Build history of the part. All positions in model axes, mm. Face numbers are marked on the shaded views. A direction names the side the tool comes from. Coordinates: 2 decimals unless noted, no trailing zeros. Order: outer loops, then holes, each group sorted by start corner. A loop starts at its lowest first (then second) coordinate and runs counter-clockwise, first axis right, second up. Notation, with made-up numbers: (21, 57.25) - (27, 57.25) arc R31 ccw to (27, 95.25) - close; hole circle Ø2 at (26, 12). An arc over 180 degrees is marked (long way). Return JSON: item names as keys, results as strings.
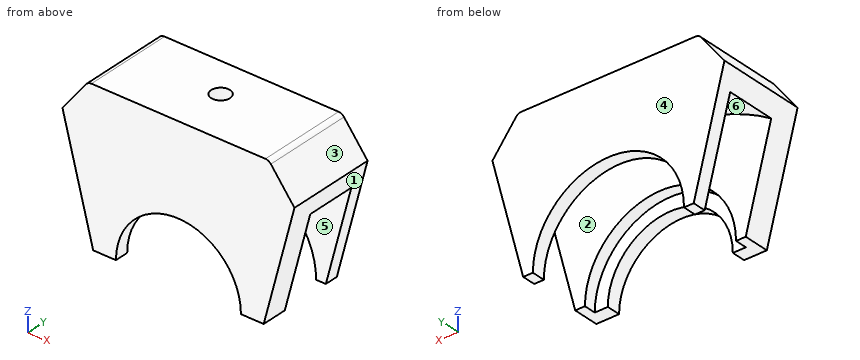
from build123d import *

# Parameters (mm, degrees)
PAD040_DEPTH            = 7.3
BODY031_PLACEMENT_ANGLE = 90
PAD042_DEPTH            = 13
SKETCH139_R             = 11
POCKET086_DEPTH         = 11
SKETCH140_R             = 9.1
POCKET087_DEPTH         = 5
SKETCH141_R             = 1.375
POCKET088_DEPTH         = 5
CHAMFER021_SIZE         = 5
FILLET005_R             = 1


with BuildPart() as obj1:
    # Sketch132 → Pad040 (new body)
    with BuildSketch(Plane.XY):
        with BuildLine():
            ThreePointArc((30, -7.93752), (0, 18.8989421975), (-30, -7.93752))
            Line((-30, -7.93752), (30, -7.93752))
        make_face()
    extrude(amount=PAD040_DEPTH)


with BuildPart() as obj1_1:
    # Body031 placement: moved
    add(obj1.part.moved(Location((0, -1.95, 0))).rotate(Axis((0, -1.95, 0), (1, 0, 0)), BODY031_PLACEMENT_ANGLE))


with BuildPart() as grip_superior:
    # Sketch138 → Pad042 (new body)
    with BuildSketch(Plane.XZ):
        Polygon((-12.413768, 0), (12.413768, 0), (18.157619, 22), (-18.157619, 22), align=None)
    extrude(amount=PAD042_DEPTH)

    # Sketch139 (on Face5 of Pad042) → Pocket086 (cut)
    with BuildSketch(Plane(origin=(0, 0, 0), x_dir=(1, 0, 0), z_dir=(0, 1, 0))):
        Circle(SKETCH139_R)
    extrude(amount=-POCKET086_DEPTH, mode=Mode.SUBTRACT)

    # Sketch140 (on Face6 of Pocket086) → Pocket087 (cut)
    with BuildSketch(Plane.XZ.offset(13)):
        Circle(SKETCH140_R)
    extrude(amount=-POCKET087_DEPTH, mode=Mode.SUBTRACT)

    # Boolean: cut obj1
    add(obj1_1.part, mode=Mode.SUBTRACT)

    # Sketch141 (on Face6 of Boolean) → Pocket088 (cut)
    with BuildSketch(Plane.XY.offset(22)):
        with Locations((0, -5.5)):
            Circle(SKETCH141_R)
    extrude(amount=-POCKET088_DEPTH, mode=Mode.SUBTRACT)

    # Chamfer021
    chamfer021_edges = [grip_superior.edges().sort_by_distance(p)[0] for p in [
        (-18.157619, -6.5, 22),
        (18.157619, -6.5, 22),
    ]]
    chamfer(chamfer021_edges, length=CHAMFER021_SIZE)

    # Fillet005
    fillet005_edges = [grip_superior.edges().sort_by_distance(p)[0] for p in [
        (-13.157619, -6.5, 22),
        (13.157619, -6.5, 22),
    ]]
    fillet(fillet005_edges, radius=FILLET005_R)


solid = grip_superior.part
1. Drop flat-ended pins along their axis: pin 1 (3.5 mm diameter, centred on x = -1.5, z = 6.5, fed in from +Y); pin 2 (1.5 mm diameter, centred on x = -1.5, y = -4.5, fed in from -Z) (3 decimals); pin 3 (3 mm diameter, centred on x = -1, y = -9, fed in from -Z); pin 4 (2 mm diameter, centred on x = 9.5, y = -5.5, fed in from -Z). Give the stop position or say it passes through.
Check values:
{"pin 1": "through", "pin 2": "z = 18.815", "pin 3": "z = 10.72", "pin 4": "z = 17.01"}
2. Cut at C-C on z = 18.5. Give the cut face in (x, y), plus the area to 3 significant figures.
Check values:
{"outline": "(-15.86, -13) - (15.86, -13) - (15.86, 0) - (-15.86, 0) - close; hole (-4.89, -9.25) - (4.89, -9.25) - (4.89, -1.95) - (-4.89, -1.95) - close", "area": "341 mm²"}
3. Cut at D-D on y = -3. Give the cut face in (x, z), plus the area to 3 significant figures.
Check values:
{"outline": "(-16.89, 17.16) - (-16.13, 14.23) arc R30.19 cw to (16.13, 14.23) - (16.89, 17.16) - (13.46, 21.61) arc R1 ccw to (12.67, 22) - (-12.67, 22) arc R1 ccw to (-13.46, 21.61) - close", "area": "140 mm²"}
4. Tool access for the marked faces 1 and 2: list every direction of +Z, -Z, +X, -X, +Y, -Y with a clear straight run to the whole face (end or side of a thin tool).
Check values:
{"face 1": "-Z, +X, +Y, -Y", "face 2": "-Z"}
5. Cut at B-B on x = 0. Give the cut face in (y, z) (3 decimals).
Check values:
{"outline": "(-13, 9.1) - (-11, 9.1) - (-11, 11) - (-9.25, 11) - (-9.25, 18.899) - (-6.875, 18.899) - (-6.875, 22) - (-13, 22) - close; (-4.125, 18.899) - (-1.95, 18.899) - (-1.95, 11) - (0, 11) - (0, 22) - (-4.125, 22) - close"}
6. Probe L1, parallel to Y at x = 0, z = 19.9 (3 decimals); L2, parallel to Y at x = 4, z = 11; L3, parallel to X at y = -5.5, z = 20.1 (3 decimals). List the from-to ranges inside material, lowest first.
Check values:
{"L1": "-13 to -6.875, -4.125 to 0", "L2": "-13 to -9.25, -1.95 to 0", "L3": "-14.625 to -1.375, 1.375 to 14.625"}
7. Mould opens along Y. For the marked faces 3, 4, 5 and 6 say: pulls with the +Y half, pulls with the -Y half, needs draft (parallel to the pull), parting line crosses it, or undercut.
Check values:
{"face 3": "needs draft", "face 4": "pulls with the +Y half", "face 5": "undercut", "face 6": "undercut"}
8. Cut at A-A on y = -5.5. Give the cut face in (x, z) (3 decimals).
Check values:
{"outline": "(-16.895, 17.162) - (-16.129, 14.229) arc R30.186 cw to (-1.375, 18.868) - (-1.375, 22) - (-12.666, 22) arc R1 ccw to (-13.458, 21.611) - close; (1.375, 18.868) arc R30.186 cw to (16.129, 14.229) - (16.895, 17.162) - (13.458, 21.611) arc R1 ccw to (12.666, 22) - (1.375, 22) - close"}
